Can you work these out from the model? Positions are in its coordinate system, mm. A direction names the side the tool comes from. Coordinates: 2 decimals unless noted, no trailing zeros. Loops run counter-clockwise (first coordinate to the right, second up) from the corner with the lowest first, then second, coordinate; pieces in that order, holes last. Notation, with made-up numbers: (-32.75, 15) -> (1.25, 15) arc R27 ccw to (1.25, 54) -> close; hole circle Ø2 at (-34, 55.5). An arc over 180 degrees is marked (long way). Use one line per item in the form item = value. Start each with the question number.
(1) Thinking about a two-plate mould opening in Z: for faces 1 (the cylindrical face through (-55.431, 7.826, 42.503)), 2 (the cylindrical face through (-14.274, 3.131, 0.628)), 3 (the flat face through (0, 25.4, 4)), which applies, released by +Z, released by -Z, zero draft, split by the parting line, or undercut?
(2) Imagine slicing it at C-C (x = 5). List the corners of the cut face in (y, z) for me (3 decimals).
(3) Imagine slicing it at B-B (y = 13). List the corners of the cut face in (x, z) for me, plus the area to 3 significant figures.
(4) Imagine slicing it at A-A (y = 3.5). State how many separate pieces and enclosed holes the cut face has, plus the area to 3 significant figures.
(5) Imagine slicing it at D-D (z = 59). List the corners of the cut face in (x, y) for me (3 decimals), plus the area to 3 significant figures.
(6) On a 3-axis mill with a long thin cutter (end or side, diameter ignored), from which of +Z, -Z, +X, -X, +Y, -Y can I reach the whole of each face in a straight line? I mean faces 4 (the cylindrical face through (-2.728, 20.571, -20.777)), 5 (the flat face through (2, 6.35, 0)), 6 (the flat face through (30, 0, 30)). Say none if no direction works.
(7) I need wall thicknesses on line 1 (Z direction, x = 0, y = 13.25); line 2 (Y direction, x = 48.5, z = -2.5) (3 decimals); line 3 (X direction, y = 14.75, z = 1.5). Which ranges of each line are inside material? Lowest first, please. Write a range as [from, to].
(8) I'm going to push flat-ended pins straight in: pin 1 (8 mm diameter, centred on x = 10.5, y = 18, fed in from -Z); pin 2 (3 mm diameter, centred on y = 19, z = 23.5, fed in from -X); pin 3 (6 mm diameter, centred on x = 10, z = -50.5, fed in from +Y) (3 decimals); pin 4 (4 mm diameter, centred on x = -4, y = 5.5, fed in from -Z). Where does each tip first touch, or does it pass through?
```python
from build123d import *

# Parameters (mm, degrees)
SKETCH1_R           = 69.85
BOSS_EXTRUDE1_DEPTH = 15.875
SKETCH2_R           = 20.955
BOSS_EXTRUDE2_DEPTH = 9.525
SKETCH13_R          = 41.275
SKETCH13_R_2        = 33.02
SKETCH13_R_3        = 25.4
SKETCH13_R_4        = 14.2875
SKETCH13_R_5        = 7.62
CUT_EXTRUDE10_DEPTH = 6.35
SKETCH14_R          = 1.190625
CUT_EXTRUDE11_DEPTH = 20.05


with BuildPart() as part:
    # Sketch1 → Boss-Extrude1 (new body)
    with BuildSketch(Plane(origin=(0, 0, 0), x_dir=(1, 0, 0), z_dir=(0, 1, 0))):
        Circle(SKETCH1_R)
    extrude(amount=BOSS_EXTRUDE1_DEPTH)

    # Sketch2 → Boss-Extrude2 (add)
    with BuildSketch(Plane(origin=(0, 15.875, 0), x_dir=(1, 0, 0), z_dir=(0, 1, 0))):
        Circle(SKETCH2_R)
    extrude(amount=BOSS_EXTRUDE2_DEPTH)

    # Sketch13 → Cut-Extrude10 (cut)
    with BuildSketch(Plane.XZ):
        Circle(SKETCH13_R)
        Circle(SKETCH13_R_2, mode=Mode.SUBTRACT)
        Circle(SKETCH13_R_3)
        Circle(SKETCH13_R_4, mode=Mode.SUBTRACT)
        Circle(SKETCH13_R_5)
    extrude(amount=-CUT_EXTRUDE10_DEPTH, mode=Mode.SUBTRACT)

    # Sketch14 → Cut-Extrude11 (cut, through all)
    with BuildSketch(Plane.XZ.offset(-6.35)):
        Circle(SKETCH14_R)
    extrude(amount=-CUT_EXTRUDE11_DEPTH, mode=Mode.SUBTRACT)


solid = part.part
```
Worked out:
q1.face_1 = split by the parting line
q1.face_2 = undercut
q1.face_3 = zero draft
q2.outline = (0, -69.671) -> (15.875, -69.671) -> (15.875, -20.35) -> (25.4, -20.35) -> (25.4, 20.35) -> (15.875, 20.35) -> (15.875, 69.671) -> (0, 69.671) -> (0, 40.971) -> (6.35, 40.971) -> (6.35, 32.639) -> (0, 32.639) -> (0, 24.903) -> (6.35, 24.903) -> (6.35, 13.384) -> (0, 13.384) -> (0, 5.75) -> (6.35, 5.75) -> (6.35, -5.75) -> (0, -5.75) -> (0, -13.384) -> (6.35, -13.384) -> (6.35, -24.903) -> (0, -24.903) -> (0, -32.639) -> (6.35, -32.639) -> (6.35, -40.971) -> (0, -40.971) -> close
q3.outline = circle Ø139.7 at (0, 0); hole circle Ø2.38 at (0, 0)
q3.area = 15,300 mm2
q4.separate_pieces = 3
q4.enclosed_holes = 3
q4.area = 11,800 mm2
q5.outline = (-37.39, 0) -> (37.39, 0) -> (37.39, 15.875) -> (-37.39, 15.875) -> close
q5.area = 1,190 mm2
q6.face_4 = +Y
q6.face_5 = -Y
q6.face_6 = +Z, -Z, +X, -X, -Y
q7.line_1 = [-69.85, -1.19], [1.19, 69.85]
q7.line_2 = [0, 15.875]
q7.line_3 = [-69.83, 69.83]
q8.pin_1 = -69.49
q8.pin_2 = through
q8.pin_3 = 15.875
q8.pin_4 = -69.82
